from build123d import *

# Parameters (mm, degrees)
SKETCH1_R           = 1.5
SKETCH1_R_2         = 1.25
BOSS_EXTRUDE1_DEPTH = 2.5


with BuildPart() as part:
    # Sketch1 → Boss-Extrude1 (new body)
    with BuildSketch(Plane(origin=(0, 0, 0), x_dir=(0, 0, -1), z_dir=(1, 0, 0))):
        with BuildLine():
            Line((-7, 10), (-7, 96))
            ThreePointArc((-7, 96), (0, 103), (7, 96))
            Line((7, 96), (7, 10))
            Line((7, 10), (-7, 10))
        make_face()
        with Locations((0, 96)):
            Circle(SKETCH1_R, mode=Mode.SUBTRACT)
        with Locations((0, 15)):
            Circle(SKETCH1_R_2, mode=Mode.SUBTRACT)
        with Locations((0, 20)):
            Circle(SKETCH1_R_2, mode=Mode.SUBTRACT)
        with Locations((0, 25)):
            Circle(SKETCH1_R_2, mode=Mode.SUBTRACT)
        with Locations((0, 30)):
            Circle(SKETCH1_R_2, mode=Mode.SUBTRACT)
    extrude(amount=BOSS_EXTRUDE1_DEPTH)


solid = part.part
Work out the finished part from the listing and answer in its coordinate system (mm). Coordinates: 2 decimals unless noted, no trailing zeros. Order: outer loops, then holes, each group sorted by start corner. A loop starts at its lowest first (then second) coordinate and runs counter-clockwise, first axis right, second up. Notation, with made-up numbers: (76, -6.5) - (123, -6.5) arc R15 cw to (123, 11.5) - close; hole circle Ø10 at (71, 76.25). An arc over 180 degrees is marked (long way). Put each result on its own line as item: value. Start each with the question number.
1) Find section A-A (y = 20). Give the vertices of the cut face in (x, z).
2) Find the intervals of material crossed by line 1 (Y direction, x = 1.3, z = 0); line 2 (Z direction, x = 1.35, y = 15.5); line 3 (Z direction, x = 2.1, y = 99), in increasing order. Write a range as from..to.
3) Find section C-C (z = 0). Give the vertices of the cut face in (x, y).
4) Find section B-B (x = 1.95). Give the vertices of the cut face in (y, z), plus the area to 3 significant figures.
5) Find section D-D (z = -6). Give the vertices of the cut face in (x, y), plus the area to 3 significant figures.
6) For a pull along Y with two mould halves and no side action, classify faces 1 (the cylindrical face through (1, 103, 0)), 2 (the flat face through (1, 54, -7)), 3 (the cylindrical face through (1.23, 18.78, 0.27)) as released by +Y, released by -Y, zero draft, split by the parting line, or undercut.
Results list:
1. outline: (0, -7) - (2.5, -7) - (2.5, -1.25) - (0, -1.25) - close; (0, 1.25) - (2.5, 1.25) - (2.5, 7) - (0, 7) - close
2. line 1: y = 10..13.75, 16.25..18.75, 21.25..23.75, 26.25..28.75, 31.25..94.5, 97.5..103
2. line 2: z = -7..-1.15, 1.15..7
2. line 3: z = -6.32..6.32
3. outline: (0, 10) - (2.5, 10) - (2.5, 13.75) - (0, 13.75) - close; (0, 16.25) - (2.5, 16.25) - (2.5, 18.75) - (0, 18.75) - close; (0, 21.25) - (2.5, 21.25) - (2.5, 23.75) - (0, 23.75) - close; (0, 26.25) - (2.5, 26.25) - (2.5, 28.75) - (0, 28.75) - close; (0, 31.25) - (2.5, 31.25) - (2.5, 94.5) - (0, 94.5) - close; (0, 97.5) - (2.5, 97.5) - (2.5, 103) - (0, 103) - close
4. outline: (10, -7) - (96, -7) arc R7 ccw to (96, 7) - (10, 7) - close; hole circle Ø2.5 at (15, 0); hole circle Ø2.5 at (20, 0); hole circle Ø2.5 at (25, 0); hole circle Ø2.5 at (30, 0); hole circle Ø3 at (96, 0)
4. area: 1,250 mm^2
5. outline: (0, 10) - (2.5, 10) - (2.5, 99.61) - (0, 99.61) - close
5. area: 224 mm^2
6. face 1: released by +Y
6. face 2: zero draft
6. face 3: undercut
